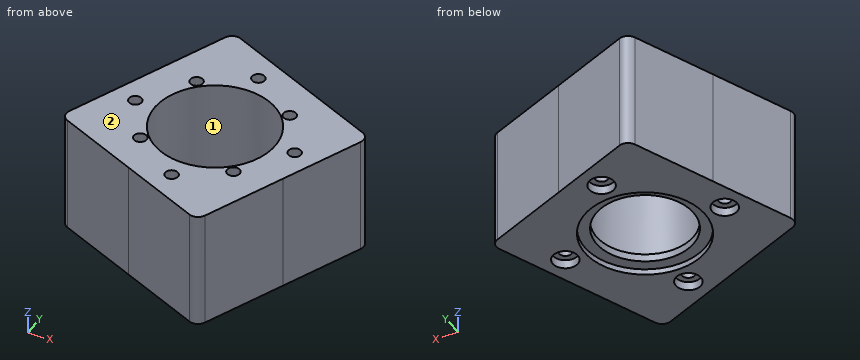
from build123d import *

# Parameters (mm, degrees)
ESQUISSE1_R                                        = 50
BOSS_EXTRU_1_DEPTH                                 = 61
ESQUISSE2_R                                        = 31
ENL_V_MAT_EXTRU_1_DEPTH                            = 72
CHAMBRAGE_POUR_VIS_T_TE_RONDE_BOMB_E_M_D           = 6.6
CHAMBRAGE_POUR_VIS_T_TE_RONDE_BOMB_E_M_CBORE_D     = 13
CHAMBRAGE_POUR_VIS_T_TE_RONDE_BOMB_E_M_CBORE_DEPTH = 4.6
D_GAGEMENT_M61_D                                   = 6.6
D_GAGEMENT_M61_DEPTH                               = 5
D_GAGEMENT_M61_TIP                                 = 1.905255888
BOSS_EXTRU_2_START                                 = -61
BOSS_EXTRU_2_DEPTH                                 = 61
ESQUISSE23_R                                       = 31
ESQUISSE23_R_2                                     = 25
BOSS_EXTRU_3_DEPTH                                 = 7
ESQUISSE24_R                                       = 31
ENL_V_MAT_EXTRU_2_DEPTH                            = 3


with BuildPart() as part:
    # Esquisse1 → Boss.-Extru.1 (new body)
    with BuildSketch(Plane.XY):
        with Locations(Location((0, 0, 0), (0, 0, 180))):
            Circle(ESQUISSE1_R)
    extrude(amount=BOSS_EXTRU_1_DEPTH)

    # Esquisse2 → Enlèv. mat.-Extru.1 (cut)
    with BuildSketch(Plane(origin=(0, 0, 0), x_dir=(-1, 0, 0), z_dir=(0, 0, -1))):
        Circle(ESQUISSE2_R)
    extrude(amount=-ENL_V_MAT_EXTRU_1_DEPTH, mode=Mode.SUBTRACT)

    # Chambrage pour vis à tête ronde bombée M61 (through all)
    with Locations(Plane(origin=(0, 0, 0), x_dir=(-1, 0, 0), z_dir=(0, 0, -1))):
        with Locations((41.25, 0), (0, 41.25), (-41.25, 0), (0, -41.25)):
            CounterBoreHole(CHAMBRAGE_POUR_VIS_T_TE_RONDE_BOMB_E_M_D / 2, CHAMBRAGE_POUR_VIS_T_TE_RONDE_BOMB_E_M_CBORE_D / 2, CHAMBRAGE_POUR_VIS_T_TE_RONDE_BOMB_E_M_CBORE_DEPTH)

    # Dégagement M61
    with Locations(Plane.XY.offset(61)):
        with Locations((-23.608593004, 25.838621023), (-25.838621023, -23.608593004), (23.608593004, -25.838621023), (25.838621023, 23.608593004)):
            Hole(D_GAGEMENT_M61_D / 2, depth=D_GAGEMENT_M61_DEPTH)
            with Locations((0, 0, -(D_GAGEMENT_M61_DEPTH + D_GAGEMENT_M61_TIP / 2))):  # 120° drill point
                Cone(0, D_GAGEMENT_M61_D / 2, D_GAGEMENT_M61_TIP, mode=Mode.SUBTRACT)

    # Esquisse20 → Boss.-Extru.2 (add)
    with BuildSketch(Plane(origin=(0, 0, 0), x_dir=(-1, 0, 0), z_dir=(0, 0, -1)).offset(BOSS_EXTRU_2_START)):
        with BuildLine():
            Line((45.900985342, 19.826738123), (28.056919844, 61.137625476))
            ThreePointArc((28.056919844, 61.137625476), (25.31054896, 63.802603508), (21.484147447, 63.74505007))
            Line((21.484147447, 63.74505007), (-19.826738428, 45.900985211))
            ThreePointArc((-19.826738428, 45.900985211), (18.437276869, 46.476519036), (45.900985342, 19.826738123))
        make_face()
        with BuildLine():
            Line((63.74505007, -21.484147447), (45.900985342, 19.826738123))
            ThreePointArc((45.900985342, 19.826738123), (46.47651917, -18.437276529), (19.826739099, -45.900984921))
            Line((19.826739099, -45.900984921), (61.137625476, -28.056919844))
            ThreePointArc((61.137625476, -28.056919844), (63.802603508, -25.31054896), (63.74505007, -21.484147447))
        make_face()
        with BuildLine():
            ThreePointArc((-45.900984787, -19.82673941), (-46.476519294, 18.437276217), (-19.826738428, 45.900985211))
            Line((-19.826738428, 45.900985211), (-61.137625476, 28.056919844))
            ThreePointArc((-61.137625476, 28.056919844), (-63.802603508, 25.31054896), (-63.74505007, 21.484147447))
            Line((-63.74505007, 21.484147447), (-45.900984787, -19.82673941))
        make_face()
        with BuildLine():
            Line((-21.484147447, -63.74505007), (19.826739099, -45.900984921))
            ThreePointArc((19.826739099, -45.900984921), (-18.437275878, -46.476519429), (-45.900984787, -19.82673941))
            Line((-45.900984787, -19.82673941), (-28.056919844, -61.137625476))
            ThreePointArc((-28.056919844, -61.137625476), (-25.31054896, -63.802603508), (-21.484147447, -63.74505007))
        make_face()
    extrude(amount=BOSS_EXTRU_2_DEPTH)

    # Esquisse23 → Boss.-Extru.3 (add)
    with BuildSketch(Plane(origin=(0, 0, 0), x_dir=(-1, 0, 0), z_dir=(0, 0, -1))):
        Circle(ESQUISSE23_R)
        Circle(ESQUISSE23_R_2, mode=Mode.SUBTRACT)
    extrude(amount=-BOSS_EXTRU_3_DEPTH)

    # Esquisse24 → Enlèv. mat.-Extru.2 (cut)
    with BuildSketch(Plane(origin=(0, 0, 0), x_dir=(-1, 0, 0), z_dir=(0, 0, -1))):
        Circle(ESQUISSE24_R)
    extrude(amount=-ENL_V_MAT_EXTRU_2_DEPTH, mode=Mode.SUBTRACT)


solid = part.part
Model file for the job. Use its own axes, mm. Face numbers are marked on the shaded views. Give positions to 0.01 mm unless a question says otherwise; leave off trailing zeros. Order: outer loops, then holes, each group sorted by start corner. A loop starts at its lowest first (then second) coordinate and runs counter-clockwise, first axis right, second up. Notation, with made-up numbers: M -29,33.25 L -15,33.25 A21 cw -15,55.25 Z; hole C 48,-3.75 d4. An arc over 180 degrees is marked long. Put each result on its own line as item: value. Start each with the question number.
(1) Band-saw the part on C-C on z = 16. Give the cut face in (x, y), then the cut area to 3 significant figures.
(2) Band-saw the part on D-D on x = 0. Count the separate pieces of the cut face and the enclosed holes in it, then the cut area to 3 significant figures.
(3) Pin check, flat tips, straight feed: pin 1 Ø11.5 at (x, y) = (-41.25, 0) entering from -Z; pin 2 Ø8 at (x, y) = (20, 10) entering from +Z; pin 3 Ø10 at (x, z) = (-42.5, 7) entering from +Y; pin 4 Ø18.5 at (x, y) = (7.5, -11) entering from -Z. Stop position of each tip, or through.
(4) Band-saw the part on A-A on y = 41.25. Give the cut face in (x, z).
(5) Band-saw the part on B-B on x = 41.25. Give the cut face in (y, z).
(6) Drill centre lines: L1, parallel to Y at x = 0, z = 1.35; L2, parallel to Y at x = -10, z = 43.5; L3, parallel to Y at x = 3.5, z = 44.5. Where is each one in solid material? Low to high. Write a range as [from, to].
(7) Pull direction X, two halves, no side cores. Call the marked faces 1 and 2: released by +X, released by -X, zero draft, split by the parting line, or undercut.
Results below:
1. outline: M -63.75,-21.48 A5 ccw -61.14,-28.06 L 21.48,-63.75 A5 ccw 28.06,-61.14 L 63.75,21.48 A5 ccw 61.14,28.06 L -21.48,63.75 A5 ccw -28.06,61.14 Z; hole C -41.25,0 d6.6; hole C 0,0 d62; hole C 0,-41.25 d6.6; hole C 0,41.25 d6.6; hole C 41.25,0 d6.6
1. area: 6,820 mm2
2. separate pieces: 4
2. enclosed holes: 0
2. area: 2,050 mm2
3. pin 1: stops at z = 4.6
3. pin 2: stops at z = 7
3. pin 3: stops at y = 39.28
3. pin 4: passes through
4. outline: M -36.65,0 L -6.5,0 L -6.5,4.6 L -3.3,4.6 L -3.3,61 L -36.65,61 Z; M 3.3,4.6 L 6.5,4.6 L 6.5,0 L 30.59,0 L 30.59,61 L 3.3,61 Z
5. outline: M -30.59,0 L -6.5,0 L -6.5,4.6 L -3.3,4.6 L -3.3,61 L -30.59,61 Z; M 3.3,4.6 L 6.5,4.6 L 6.5,0 L 36.65,0 L 36.65,61 L 3.3,61 Z
6. L1: y = [-54.47, -47.75], [-34.75, -31], [31, 34.75], [47.75, 54.47]
6. L2: y = [-50.15, -29.34], [29.34, 58.78]
6. L3: y = [-55.98, -30.8], [30.8, 52.95]
7. face 1: undercut
7. face 2: zero draft
